Build history of the part. All positions in model axes, mm. Face numbers are marked on the shaded views. A direction names the side the tool comes from. Coordinates: 2 decimals unless noted, no trailing zeros. Loops run counter-clockwise (first coordinate to the right, second up) from the corner with the lowest first, then second, coordinate; pieces in that order, holes last. Notation, with made-up numbers: (62, 67) -> (94, 67) arc R19 ccw to (94, 80) -> close; hole circle Ø9 at (-9.5, 61.25). An arc over 180 degrees is marked (long way). One line per item, written item: value. Start each with the question number.
```python
from build123d import *

# Parameters (mm, degrees)
BOSS_EXTRUDE1_DEPTH = 20
FILLET1_R           = 2


with BuildPart() as part:
    # Sketch1 → Boss-Extrude1 (new body)
    with BuildSketch(Plane.XY):
        Polygon((0, 0), (90, 0), (66.905989232, 40), (49.585481157, 10), (20, 10), (20, 14.226497308), (30, 20), (30, 30), (0, 30), align=None)
    extrude(amount=BOSS_EXTRUDE1_DEPTH)

    # Fillet1
    fillet1_edges = [part.edges().sort_by_distance(p)[0] for p in [
        (30, 20, 10),
        (20, 14.226497308, 10),
        (20, 10, 10),
        (49.585481157, 10, 10),
        (66.905989232, 40, 10),
        (90, 0, 10),
    ]]
    fillet(fillet1_edges, radius=FILLET1_R)


solid = part.part
```
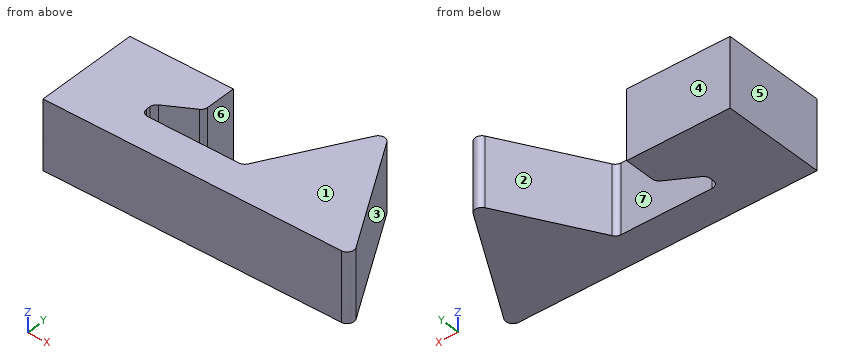
Item 1: Tool access for the marked faces 4, 5, 6 and 7: list every direction of +Z, -Z, +X, -X, +Y, -Y with a clear straight run to the whole face (end or side of a thin tool).
Item 2: Band-saw the part on C-C, the plane x = 43.5. List the corners of the cut face in (y, z), and give its area (3 significant figures).
Item 3: Drop flat-ended pins along their axis: pin 1 Ø10 at (y, z) = (24.5, 2.5) entering from +X; pin 2 Ø3 at (y, z) = (10.5, 11) entering from +X; pin 3 Ø12 at (y, z) = (11.5, 7) entering from +X. Give the stop position or say it passes through.
Item 4: Probe probe 1 along Y at (x, z) = (39, 12.5); probe 2 along X at (y, z) = (6, 19); probe 3 along Y at (x, z) = (7.5, 7.5). List the from-to ranges inside material, lowest first.
Item 5: Band-saw the part on D-D, the plane y = 29. List the corners of the cut face in (x, z).
Item 6: Band-saw the part on A-A, the plane z = 15. List the corners of the cut face in (x, y), and give its area (3 significant figures).
Item 7: Two-plate mould, pull along X, no slides. Class the marked faces 1, 2 and 3: +X half, -X half, draft (parallel to the pull), parting line (faces both ways), or undercut.
Item 8: Band-saw the part on B-B, the plane y = 17. List the corners of the cut face in (x, z), and give its area (3 significant figures).
Worked out:
1. face 4: +Z, -Z, -X, +Y
1. face 5: +Z, -Z, -X, +Y, -Y
1. face 6: +Z, -Z, +Y
1. face 7: +Z, -Z
2. outline: (0, 0) -> (10, 0) -> (10, 20) -> (0, 20) -> close
2. area: 200 mm²
3. pin 1: stops at x = 78.74
3. pin 2: stops at x = 84.8
3. pin 3: stops at x = 86.82
4. probe 1: y = 0 to 10
4. probe 2: x = 0 to 86.54
4. probe 3: y = 0 to 30
5. outline: (0, 0) -> (30, 0) -> (30, 20) -> (0, 20) -> close; (60.56, 0) -> (73.26, 0) -> (73.26, 20) -> (60.56, 20) -> close
6. outline: (0, 0) -> (86.54, 0) arc R2 ccw to (88.27, 3) -> (68.64, 37) arc R2 ccw to (65.17, 37) -> (50.16, 11) arc R2 cw to (48.43, 10) -> (22, 10) arc R2 cw to (20, 12) -> (20, 13.07) arc R2 cw to (21, 14.8) -> (29, 19.42) arc R2 ccw to (30, 21.15) -> (30, 30) -> (0, 30) -> close
6. area: 1,920 mm²
7. face 1: draft
7. face 2: undercut
7. face 3: +X half
8. outline: (0, 0) -> (24.8, 0) -> (24.8, 20) -> (0, 20) -> close; (53.63, 0) -> (80.19, 0) -> (80.19, 20) -> (53.63, 20) -> close
8. area: 1,030 mm²
